Could you check a few things on this model? Use its own coordinates, in mm. Round coordinates to 2 decimals unless told otherwise and drop trailing zeros. Order: outer loops, then holes, each group sorted by start corner. A loop starts at its lowest first (then second) coordinate and runs counter-clockwise, first axis right, second up. Notation, with made-up numbers: M -26,62 L -14,62 A10 ccw -14,77 Z; hole C 3.5,84 d10. An arc over 180 degrees is marked long. Write each question's results on one line, items separated by ' | '. Start each with the question number.
1. I'm going to push flat-ended pins straight in: pin 1 (2 mm diameter, centred on y = 490.5, z = -17.5, fed in from +X); pin 2 (6 mm diameter, centred on x = -19, z = -11, fed in from +Y). Where does each tip first touch, or does it pass through?
2. Please list where these lines run through material, in increasing order: L1, parallel to Z at x = -19, y = 569 (3 decimals); L2, parallel to Y at x = -2.5, z = -10.75.
3. Suppose I cut it at B-B on x = -13.5. Write out the boundary of the cut face in (y, z) (3 decimals), and give its area (3 significant figures).
4. Suppose I cut it at C-C on y = 82.5. Write out the boundary of the cut face in (x, z) (3 decimals).
5. Suppose I cut it at A-A on z = -13.5. Write out the boundary of the cut face in (x, y) (3 decimals).
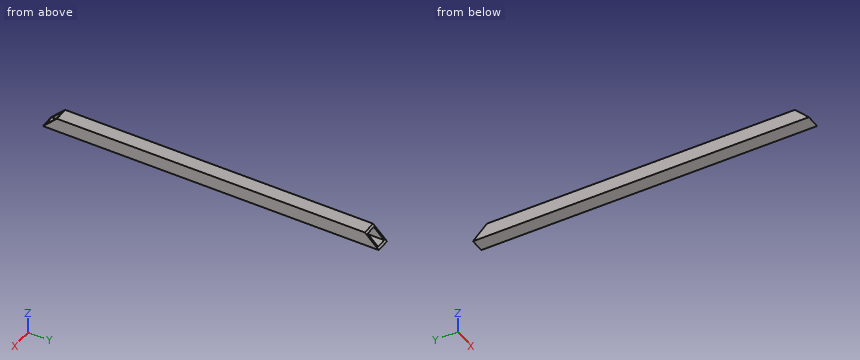
Autodesk Inventor part; units mm, degrees
ref_plane "YZ Plane" through (0, 0, 0) normal (1, 0, 0) x (0, 1, 0)
ref_plane "XZ Plane" through (0, 0, 0) normal (0, 1, 0) x (-1, 0, 0)
ref_plane "XY Plane" through (0, 0, 0) normal (0, 0, 1) x (1, 0, 0)
sketch "Sketch1" plane through (0, 0, 0) normal (0, 1, 0) x (-1, 0, 0)
  line L0 (0, 0) -> (25.4, 0)
  line L1 (25.4, 0) -> (25.4, -25.4)
  line L2 (25.4, -25.4) -> (0, -25.4)
  line L3 (0, -25.4) -> (0, 0)
  line L4 (3.175, -3.175) -> (22.225, -3.175)
  line L5 (22.225, -3.175) -> (22.225, -22.225)
  line L6 (22.225, -22.225) -> (3.175, -22.225)
  line L7 (3.175, -22.225) -> (3.175, -3.175)
  dimension "d0" = 25.4
  dimension "d1" = 25.4
  dimension "d2" = 3.175
extrude "Extrusion1" add sketch "Sketch1" along normal blind 609.6
chamfer "Chamfer1" distance 25.4 angle 45 2 edges at (-12.7, 609.6, 0) (-12.7, 0, 0)
properties part number "1x1x24"
Filled sheet:
1) pin 1: stops at x = 0 | pin 2: passes through
2) L1: z = -25.4 to -22.225, -3.175 to 0 | L2: y = 14.65 to 594.95
3) outline: M 0,-25.4 L 609.6,-25.4 L 606.425,-22.225 L 3.175,-22.225 Z; M 22.225,-3.175 L 587.375,-3.175 L 584.2,0 L 25.4,0 Z | area: 3,710 mm^2
4) outline: M -25.4,-25.4 L 0,-25.4 L 0,0 L -25.4,0 Z; hole M -22.225,-22.225 L -3.175,-22.225 L -3.175,-3.175 L -22.225,-3.175 Z
5) outline: M -25.4,11.9 L -22.225,11.9 L -22.225,597.7 L -25.4,597.7 Z; M -3.175,11.9 L 0,11.9 L 0,597.7 L -3.175,597.7 Z
